Design review of the part shown in the three views and the two pictorial views. Dimensions are in mm from the part's minimum x, y and z. A direction names the side the tool comes from. Round coordinates to 2 decimals unless told otherwise and drop trailing zeros. Write each loop counter-clockwise with the first axis right and the second up, starting at its lowest first coordinate (ties: lowest second). Pieces come first, ordered by that corner, then holes. Notation, with made-up numbers: (-19, 89.5) -> (4, 89.5) arc R23 ccw to (4, 124.5) -> close; hole circle Ø9 at (-33.75, 33). An arc over 180 degrees is marked (long way). Return JSON: item names as keys, results as strings. Group by question number.
1. Take a section at B-B, the plane x = 9. Write out the cut boundary in (y, z).
2. Clearance check with flat-ended pins moving along their axes: P1, Ø10, axis at x = 50, y = 9, coming from the +Z side; P2, Ø10.5, axis at x = 3.5, z = 21.5, coming from the -Y side; P3, Ø16.5, axis at x = 36, z = 61, coming from the -Y side. State where each tip first meets the part, or that it passes through.
3. Mouldability with a two-part tool opening along X and no side actions: class the marked faces 6, 7 and 8 as pulls with the +X half, pulls with the -X half, needs draft (parallel to the pull), parting line crosses it, or undercut.
4. Tool access review of the marked faces 1, 2, 3, 4 and 5: name each direction out of +Z, -Z, +X, -X, +Y, -Y from which nothing blocks a thin tool from reaching the whole face with its end or side.
5. Take a section at D-D, the plane y = 30. Write out the cut boundary in (x, z).
6. Take a section at C-C, the plane z = 12. Write out the cut boundary in (x, y), then the cut area to 3 significant figures.
7. For line 1 along Z through (x, y) = (22, 25); line 2 along Y through (x, z) = (48, 55.5); line 3 along Y through (x, z) = (59.5, 21), list the stretches that pass through material, from the lowest coordinate up. Write a range as from..to.
8. Take a section at A-A, the plane z = 80.5. Write out the cut boundary in (x, y), then the cut area to 3 significant figures.
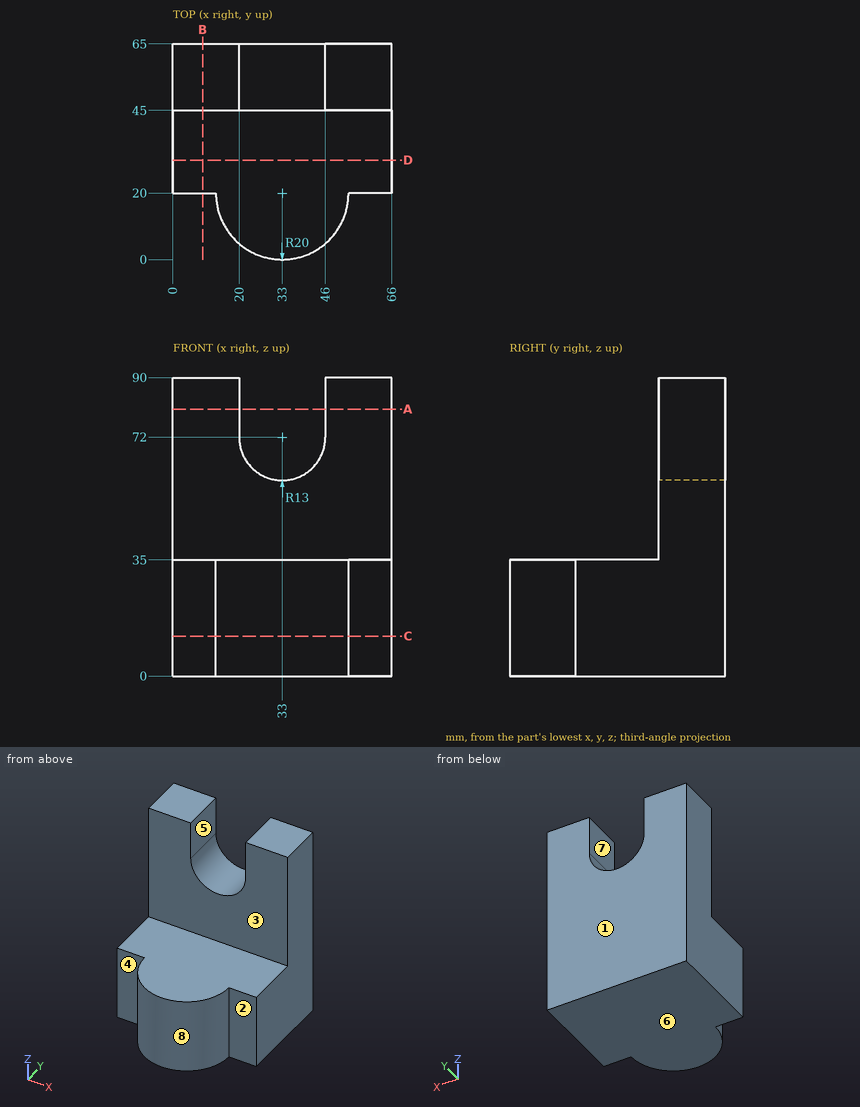
Output:
{
 "1": {"outline": "(20, 0) -> (65, 0) -> (65, 90) -> (45, 90) -> (45, 35) -> (20, 35) -> close"},
 "2": {"P1": "stops at z = 35", "P2": "stops at y = 20", "P3": "stops at y = 45"},
 "3": {"face 6": "needs draft", "face 7": "undercut", "face 8": "parting line crosses it"},
 "4": {"face 1": "+Z, -Z, +X, -X, +Y", "face 2": "+Z, -Z, +X, -Y", "face 3": "+Z, +X, -X, -Y", "face 4": "+Z, -Z, -X, -Y", "face 5": "+Z, +Y, -Y"},
 "5": {"outline": "(0, 0) -> (66, 0) -> (66, 35) -> (0, 35) -> close"},
 "6": {"outline": "(0, 20) -> (13, 20) arc R20 ccw to (53, 20) -> (66, 20) -> (66, 65) -> (0, 65) -> close", "area": "3,600 mm^2"},
 "7": {"line 1": "z = 0..35", "line 2": "y = 45..65", "line 3": "y = 20..65"},
 "8": {"outline": "(0, 45) -> (20, 45) -> (20, 65) -> (0, 65) -> close; (46, 45) -> (66, 45) -> (66, 65) -> (46, 65) -> close", "area": "800 mm^2"}
}
